```python
from build123d import *

# Parameters (mm, degrees)
BOSS_EXTRUDE1_DEPTH = 60
FILLET2_R           = 2.5
FILLET3_R           = 2.5
FILLET4_R           = 30
FILLET5_R           = 30
SKETCH3_R           = 11
SKETCH3_R_2         = 1.742420083
CUT_EXTRUDE1_DEPTH  = 5
BOSS_EXTRUDE3_START = -2
BOSS_EXTRUDE3_DEPTH = 2
BOSS_EXTRUDE4_DEPTH = 2
SKETCH7_R           = 2
CUT_EXTRUDE2_DEPTH  = 2


with BuildPart() as part:
    # Sketch2 → Boss-Extrude1 (new body)
    with BuildSketch(Plane.XY):
        with BuildLine():
            Line((0.5, 0), (63, 0))
            Line((63, 0), (63, -2))
            Line((63, -2), (0.5, -2))
            ThreePointArc((0.5, -2), (-1.267766953, -1.267766953), (-2, 0.5))
            Line((-2, 0.5), (-2, 53))
            Line((-2, 53), (0, 53))
            Line((0, 53), (0, 0.5))
            ThreePointArc((0, 0.5), (0.146446609, 0.146446609), (0.5, 0))
        make_face()
    extrude(amount=BOSS_EXTRUDE1_DEPTH)

    # Fillet2
    fillet2_edges = [part.edges().sort_by_distance(p)[0] for p in [
        (63, -1, 60),
    ]]
    fillet(fillet2_edges, radius=FILLET2_R)

    # Fillet3
    fillet3_edges = [part.edges().sort_by_distance(p)[0] for p in [
        (63, -1, 0),
    ]]
    fillet(fillet3_edges, radius=FILLET3_R)

    # Fillet4
    fillet4_edges = [part.edges().sort_by_distance(p)[0] for p in [
        (-1, 53, 60),
    ]]
    fillet(fillet4_edges, radius=FILLET4_R)

    # Fillet5
    fillet5_edges = [part.edges().sort_by_distance(p)[0] for p in [
        (-1, 53, 0),
    ]]
    fillet(fillet5_edges, radius=FILLET5_R - 0.0001)  # a hair under: the kernel refuses the full size

    # Sketch3 → Cut-Extrude1 (cut)
    with BuildSketch(Plane(origin=(0, 0, 0), x_dir=(0, 0, -1), z_dir=(1, 0, 0))):
        with Locations(Location((-30, 23, 0), (0, 0, 90))):
            Circle(SKETCH3_R)
        with Locations(Location((-39.899494937, 13.100505063, 0), (0, 0, 90))):
            Circle(SKETCH3_R_2)
        with Locations(Location((-39.899494937, 32.899494937, 0), (0, 0, 90))):
            Circle(SKETCH3_R_2)
        with Locations(Location((-20.100505063, 32.899494937, 0), (0, 0, 90))):
            Circle(SKETCH3_R_2)
        with Locations(Location((-20.100505063, 13.100505063, 0), (0, 0, 90))):
            Circle(SKETCH3_R_2)
    extrude(amount=-CUT_EXTRUDE1_DEPTH, mode=Mode.SUBTRACT)

    # Sketch4 → Boss-Extrude3 (add)
    with BuildSketch(Plane.XY.offset(60).offset(BOSS_EXTRUDE3_START)):
        with BuildLine():
            Line((0, 20.075175272), (28.67032155, 0))
            Line((28.67032155, 0), (0.5, 0))
            ThreePointArc((0.5, 0), (0.146446609, 0.146446609), (0, 0.5))
            Line((0, 0.5), (0, 20.075175272))
        make_face()
    extrude(amount=BOSS_EXTRUDE3_DEPTH)

    # Sketch6 → Boss-Extrude4 (add)
    with BuildSketch(Plane(origin=(0, 0, 0), x_dir=(-1, 0, 0), z_dir=(0, 0, -1))):
        with BuildLine():
            Line((0, 0.5), (0, 20.075175272))
            Line((0, 20.075175272), (-28.67032155, 0))
            Line((-28.67032155, 0), (-0.5, 0))
            ThreePointArc((-0.5, 0), (-0.146446609, 0.146446609), (0, 0.5))
        make_face()
    extrude(amount=-BOSS_EXTRUDE4_DEPTH)

    # Sketch7 → Cut-Extrude2 (cut)
    with BuildSketch(Plane(origin=(0, 0, 0), x_dir=(1, 0, 0), z_dir=(0, 1, 0))):
        with Locations(Location((54, -53, 0), (0, 0, 270))):
            Circle(SKETCH7_R)
        with Locations(Location((54, -7, 0), (0, 0, 270))):
            Circle(SKETCH7_R)
        with Locations(Location((10, -7, 0), (0, 0, 270))):
            Circle(SKETCH7_R)
        with Locations(Location((10, -53, 0), (0, 0, 270))):
            Circle(SKETCH7_R)
        with BuildLine():
            Line((44.5, -55), (39.5, -55))
            ThreePointArc((39.5, -55), (37.5, -53), (39.5, -51))
            Line((39.5, -51), (44.5, -51))
            ThreePointArc((44.5, -51), (46.5, -53), (44.5, -55))
        make_face()
        with BuildLine():
            Line((44.5, -9), (39.5, -9))
            ThreePointArc((39.5, -9), (37.5, -7), (39.5, -5))
            Line((39.5, -5), (44.5, -5))
            ThreePointArc((44.5, -5), (46.5, -7), (44.5, -9))
        make_face()
        with BuildLine():
            Line((24.5, -9), (19.5, -9))
            ThreePointArc((19.5, -9), (17.5, -7), (19.5, -5))
            Line((19.5, -5), (24.5, -5))
            ThreePointArc((24.5, -5), (26.5, -7), (24.5, -9))
        make_face()
        with BuildLine():
            Line((24.5, -55), (19.5, -55))
            ThreePointArc((19.5, -55), (17.5, -53), (19.5, -51))
            Line((19.5, -51), (24.5, -51))
            ThreePointArc((24.5, -51), (26.5, -53), (24.5, -55))
        make_face()
        with BuildLine():
            Line((24.79106514, -18), (24.79106514, -42))
            ThreePointArc((24.79106514, -42), (22, -44.79106514), (19.20893486, -42))
            Line((19.20893486, -42), (19.20893486, -18))
            ThreePointArc((19.20893486, -18), (22, -15.20893486), (24.79106514, -18))
        make_face()
        with BuildLine():
            Line((44.79106514, -18), (44.79106514, -42))
            ThreePointArc((44.79106514, -42), (42, -44.79106514), (39.20893486, -42))
            Line((39.20893486, -42), (39.20893486, -18))
            ThreePointArc((39.20893486, -18), (42, -15.20893486), (44.79106514, -18))
        make_face()
    extrude(amount=-CUT_EXTRUDE2_DEPTH, mode=Mode.SUBTRACT)


solid = part.part
```
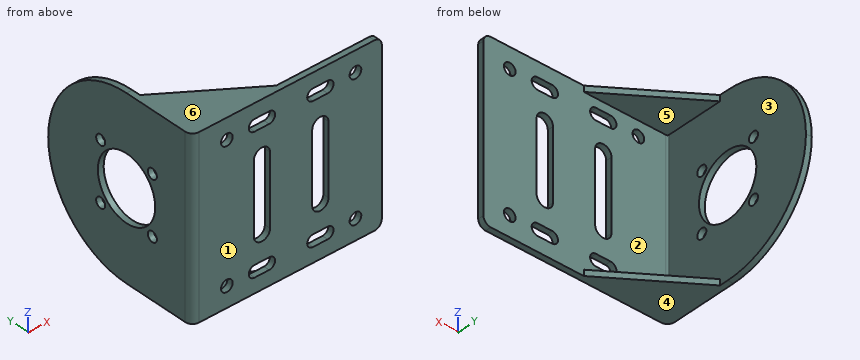
Source: CAD feature listing. Evaluate the final solid. Frame: model axes, mm. Face numbers are marked on the shaded views. A direction names the side the tool comes from. Coordinates: 2 decimals unless noted, no trailing zeros. Loops run counter-clockwise (first coordinate to the right, second up) from the corner with the lowest first, then second, coordinate; pieces in that order, holes last. Notation, with made-up numbers: (-16.5, 22.5) -> (-2.5, 22.5) arc R24 ccw to (-2.5, 56.5) -> close; hole circle Ø6 at (44, -1.75). An arc over 180 degrees is marked (long way). One line per item, written item: value. Start each with the question number.
Q1. Set-up query: the marked faces 5 and 6. Return all of +Z, -Z, +X, -X, +Y, -Y with unobstructed straight access to the full face (end or side cutting, diameter ignored); none if empty.
Q2. Section query A-A, the plane x = 42. Return the cut outline in (y, z), and give its area (3 significant figures).
Q3. Section query C-C, the plane y = 19. Return the cut outline in (x, z), and give its area (3 significant figures).
Q4. Mould query, pull axis Z, two halves, no side actions, for the marked faces 1, 2, 3 and 4. Classes: pulls with the +Z half, pulls with the -Z half, needs draft (parallel to the pull), parting line crosses it, or undercut.
Q5. Line query: line 1 along X through (y, z) = (-0.85, 7); line 2 along X through (y, z) = (3.5, 49). Output: solid intervals per line, ascending.
Q6. Section query B-B, the plane z = 24. Return the cut outline in (x, y), and give its area (3 significant figures).
Q7. Contact query for flat-ended pins moving along their axis: P1, Ø1, axis at y = -0.5, z = 29, coming from the -X side; P2, Ø3, axis at y = 32.9, z = 20.1, coming from the +X side; P3, Ø10, axis at y = 41, z = 15, coming from the +X side; P4, Ø0.6, axis at y = -1, z = 26, coming from the -X side. Output: stop coordinate, or through.
Q8. Section query D-D, the plane x = 54. Return the cut outline in (y, z).
Results:
1. face 5: +X, +Y
1. face 6: +Z, +X, -X, +Y, -Y
2. outline: (-2, 0) -> (0, 0) -> (0, 5) -> (-2, 5) -> close; (-2, 9) -> (0, 9) -> (0, 15.21) -> (-2, 15.21) -> close; (-2, 44.79) -> (0, 44.79) -> (0, 51) -> (-2, 51) -> close; (-2, 55) -> (0, 55) -> (0, 60) -> (-2, 60) -> close
2. area: 44.8 mm^2
3. outline: (-2, 0) -> (1.54, 0) -> (1.54, 2) -> (0, 2) -> (0, 19.75) -> (-2, 19.75) -> close; (-2, 40.25) -> (0, 40.25) -> (0, 58) -> (1.54, 58) -> (1.54, 60) -> (-2, 60) -> close
3. area: 85.2 mm^2
4. face 1: needs draft
4. face 2: undercut
4. face 3: undercut
4. face 4: pulls with the -Z half
5. line 1: -1.6 to 8, 12 to 17.5, 26.5 to 37.5, 46.5 to 52, 56 to 63
5. line 2: -2 to 0
6. outline: (-2, 0.5) arc R2.5 ccw to (0.5, -2) -> (19.21, -2) -> (19.21, 0) -> (0.5, 0) arc R0.5 cw to (0, 0.5) -> (0, 13.78) -> (-2, 13.78) -> close; (-2, 32.22) -> (0, 32.22) -> (0, 52.39) -> (-2, 52.39) -> close; (24.79, -2) -> (39.21, -2) -> (39.21, 0) -> (24.79, 0) -> close; (44.79, -2) -> (63, -2) -> (63, 0) -> (44.79, 0) -> close
6. area: 174 mm^2
7. P1: x = -1.95
7. P2: through
7. P3: x = 0
7. P4: x = -1.69
8. outline: (-2, 0) -> (0, 0) -> (0, 5) -> (-2, 5) -> close; (-2, 9) -> (0, 9) -> (0, 51) -> (-2, 51) -> close; (-2, 55) -> (0, 55) -> (0, 60) -> (-2, 60) -> close
